Geometry check sheet. Reference: drawing and pictorial views, mm from the part's lowest x, y, z. Give positions to 0.01 mm unless a question says otherwise; leave off trailing zeros. Loops run counter-clockwise (first coordinate to the right, second up) from the corner with the lowest first, then second, coordinate; pieces in that order, holes last. Notation, with made-up numbers: (-16.75, -11.5) -> (14.25, -11.5) arc R35 cw to (14.25, 27.5) -> close; hole circle Ø2 at (46, -36). An arc over 180 degrees is marked (long way). One line per item, written item: value. Start each with the question number.
(1) Gauge pin test, flat ends, axial feed: pin 1 Ø2 at (x, y) = (41, 6) entering from -Z; pin 2 Ø6 at (x, z) = (30.5, 2.5) entering from +Y; pin 3 Ø2 at (x, z) = (45, 10) entering from +Y; pin 4 Ø2 at (x, y) = (13.5, 9.5) entering from -Z. Record the tip position at first contact, or that the pin passes through.
(2) Draft check along Y on the marked faces 1, 2 and 3. Enter one of: pulls with the +Y half, pulls with the -Y half, needs draft (parallel to the pull), parting line crosses it, or undercut.
(3) Scan lines: line 1 along Y through (x, z) = (27.5, 14.05); line 2 along Y through (x, z) = (27.5, 9). Record each from-to range of solid material in increasing order. Write a range as from..to.
(4) Sectioned sample at D-D, the plane z = 8.25. Record the cut outline in (x, y), then the cut area to 3 significant figures.
(5) Sectioned sample at C-C, the plane x = 35. Record the cut outline in (y, z).
(6) Sectioned sample at A-A, the plane x = 27.5. Record the cut outline in (y, z), then the cut area to 3 significant figures.
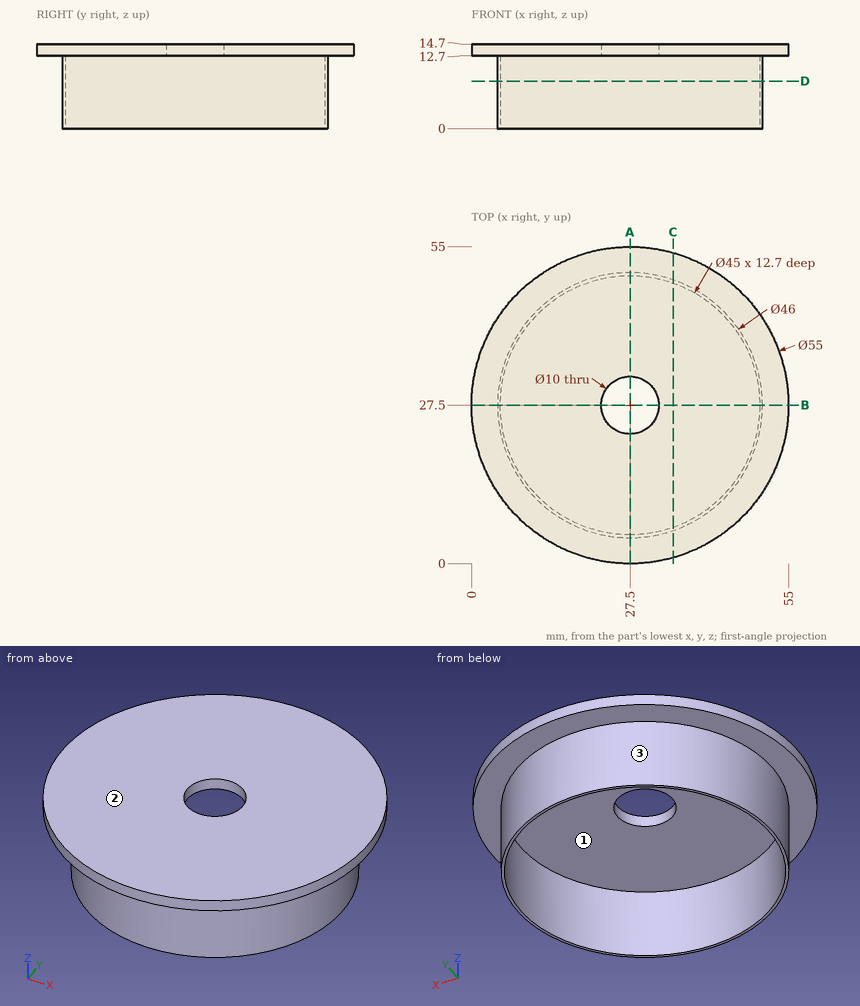
Calculated:
1. pin 1: stops at z = 12.7
1. pin 2: stops at y = 50.5
1. pin 3: stops at y = 43.52
1. pin 4: stops at z = 0
2. face 1: undercut
2. face 2: needs draft
2. face 3: parting line crosses it
3. line 1: y = 0..22.5, 32.5..55
3. line 2: y = 4.5..5, 50..50.5
4. outline: circle Ø46 at (27.5, 27.5); hole circle Ø45 at (27.5, 27.5)
4. area: 71.5 mm2
5. outline: (1.04, 12.7) -> (5.76, 12.7) -> (5.76, 0) -> (6.29, 0) -> (6.29, 12.7) -> (48.71, 12.7) -> (48.71, 0) -> (49.24, 0) -> (49.24, 12.7) -> (53.96, 12.7) -> (53.96, 14.7) -> (1.04, 14.7) -> close
6. outline: (0, 12.7) -> (4.5, 12.7) -> (4.5, 0) -> (5, 0) -> (5, 12.7) -> (22.5, 12.7) -> (22.5, 14.7) -> (0, 14.7) -> close; (32.5, 12.7) -> (50, 12.7) -> (50, 0) -> (50.5, 0) -> (50.5, 12.7) -> (55, 12.7) -> (55, 14.7) -> (32.5, 14.7) -> close
6. area: 103 mm2
